from build123d import *

# Parameters (mm, degrees)
BOSS_EXTRUDE2_DEPTH = 6
BOSS_EXTRUDE4_DEPTH = 12
CUT_EXTRUDE4_DEPTH  = 56.306509563
FILLET3_R           = 5
FILLET7_R           = 2
FILLET4_R           = 2
FILLET5_R           = 0.5
FILLET6_R           = 1


with BuildPart() as part:
    # Sketch1 → Boss-Extrude2 (new body)
    with BuildSketch(Plane(origin=(0, 0, 0), x_dir=(1, 0, 0), z_dir=(0, 1, 0))):
        Polygon((13, 5), (-13, 5), (-13, 16), (-25.45, 16), (-25.45, 0), (25.45, 0), (25.45, 16), (13, 16), align=None)
        with BuildLine():
            ThreePointArc((-19.547918472, 10.202081528), (-20.75, 7.3), (-21.952081528, 10.202081528))
            Line((-21.952081528, 10.202081528), (-20.75, 11.404163056))
            Line((-20.75, 11.404163056), (-19.547918472, 10.202081528))
        make_face(mode=Mode.SUBTRACT)
        with BuildLine():
            Line((20.75, 11.404163056), (21.952081528, 10.202081528))
            ThreePointArc((21.952081528, 10.202081528), (20.75, 7.3), (19.547918472, 10.202081528))
            Line((19.547918472, 10.202081528), (20.75, 11.404163056))
        make_face(mode=Mode.SUBTRACT)
    extrude(amount=BOSS_EXTRUDE2_DEPTH)

    # Sketch1<4> → Boss-Extrude4 (add)
    with BuildSketch(Plane(origin=(0, 0, 0), x_dir=(1, 0, 0), z_dir=(0, 1, 0))):
        Polygon((25.45, 0), (-25.45, 0), (-25.45, -18), (-20.45, -18), (-20.45, -3), (9.55, -3), (9.55, -18), (14.55, -18), (14.55, -3), (25.45, -3), align=None)
    extrude(amount=BOSS_EXTRUDE4_DEPTH)

    # Sketch9 → Cut-Extrude4 (cut, through all)
    with BuildSketch(Plane.ZY.offset(25.45)):
        with BuildLine():
            Line((9.378679656, 8.121320344), (11.5, 10.242640687))
            Line((11.5, 10.242640687), (13.621320344, 8.121320344))
            ThreePointArc((13.621320344, 8.121320344), (11.5, 3), (9.378679656, 8.121320344))
        make_face()
    extrude(amount=-CUT_EXTRUDE4_DEPTH, mode=Mode.SUBTRACT)

    # Fillet3
    fillet3_edges = [part.edges().sort_by_distance(p)[0] for p in [
        (-22.95, 12, 18),
        (12.05, 12, 18),
    ]]
    fillet(fillet3_edges, radius=FILLET3_R)

    # Fillet7
    fillet7_edges = [part.edges().sort_by_distance(p)[0] for p in [
        (-5.45, 0, 3),
    ]]
    fillet(fillet7_edges, radius=FILLET7_R)

    # Fillet4
    # the kernel refuses this fillet: 2 mm, written as the material it adds along each edge
    with BuildSketch(Plane(origin=(9.55, 2, 1), x_dir=(0, 0.8017442392976483, -0.5976672776328277), z_dir=(0, 0.5976672776328277, 0.8017442392976483))) as fillet4_piece_1_section:
        with BuildLine():
            CenterArc((2 + FILLET4_R, FILLET4_R), FILLET4_R, 180, 90)
            Line((2, FILLET4_R), (2, 0))
            Line((2, 0), (2 + FILLET4_R, 0))
        make_face()
    fillet4_piece_1 = revolve(axis=Axis((9.55, 2, 1), (-1, 0, 0)), revolution_arc=233.296989237, mode=Mode.PRIVATE)
    fillet4_piece_1 = split(fillet4_piece_1, bisect_by=Plane(origin=(8.926743459, 0, 2.499877942), z_dir=(0, 1, 0)), keep=Keep.TOP, mode=Mode.PRIVATE)
    add(fillet4_piece_1)
    with BuildSketch(Plane(origin=(-20.45, 2, 1), x_dir=(0, 0.8017442392976483, -0.5976672776328277), z_dir=(0, 0.5976672776328277, 0.8017442392976483))) as fillet4_piece_2_section:
        with BuildLine():
            CenterArc((2 + FILLET4_R, -FILLET4_R), FILLET4_R, 90, 90)
            Line((2 + FILLET4_R, 0), (2, 0))
            Line((2, 0), (2, -FILLET4_R))
        make_face()
    fillet4_piece_2 = revolve(axis=Axis((-20.45, 2, 1), (-1, 0, 0)), revolution_arc=233.296989237, mode=Mode.PRIVATE)
    fillet4_piece_2 = split(fillet4_piece_2, bisect_by=Plane(origin=(-19.826743524, 0, 2.499877995), z_dir=(0, 1, 0)), keep=Keep.TOP, mode=Mode.PRIVATE)
    add(fillet4_piece_2)
    with BuildSketch(Plane(origin=(14.55, 0, 3), x_dir=(1, 0, 0), z_dir=(0, 1, 0))) as fillet4_piece_3:
        with BuildLine():
            CenterArc((FILLET4_R, -FILLET4_R), FILLET4_R, 90, 90)
            Line((0, -FILLET4_R), (0, 0))
            Line((0, 0), (FILLET4_R, 0))
        make_face()
    extrude(amount=12)
    with BuildSketch(Plane(origin=(-20.45, 2, 3), x_dir=(1, 0, 0), z_dir=(0, 1, 0))) as fillet4_piece_4:
        with BuildLine():
            CenterArc((FILLET4_R, -FILLET4_R), FILLET4_R, 90, 90)
            Line((0, -FILLET4_R), (0, 0))
            Line((0, 0), (FILLET4_R, 0))
        make_face()
    extrude(amount=10)
    with BuildSketch(Plane(origin=(9.55, 2, 3), x_dir=(-1, 0, 0), z_dir=(0, 1, 0))) as fillet4_piece_5:
        with BuildLine():
            CenterArc((FILLET4_R, FILLET4_R), FILLET4_R, 180, 90)
            Line((0, FILLET4_R), (0, 0))
            Line((0, 0), (FILLET4_R, 0))
        make_face()
    extrude(amount=10)

    # Fillet5
    fillet5_edges = [part.edges().sort_by_distance(p)[0] for p in [
        (0, 6, 0),
    ]]
    fillet(fillet5_edges, radius=FILLET5_R)

    # Fillet6
    fillet6_edges = [part.edges().sort_by_distance(p)[0] for p in [
        (-25.45, 3, -16),
        (-13, 3, -16),
        (13, 3, -16),
        (25.45, 3, -16),
        (25.45, 6, 3),
        (-22.95, 0, 18),
        (12.05, 0, 18),
    ]]
    fillet(fillet6_edges, radius=FILLET6_R)


solid = part.part
Could you check a few things on this model? Use its own coordinates, in mm. A direction names the side the tool comes from. Give positions to 0.01 mm unless a question says otherwise; leave off trailing zeros. Write each loop counter-clockwise with the first axis right and the second up, starting at its lowest first coordinate (ties: lowest second). Pieces come first, ordered by that corner, then holes. Notation, with made-up numbers: (-33, 71.25) -> (21, 71.25) arc R25 ccw to (21, 99.25) -> close; hole circle Ø1 at (23.25, 82.25). An arc over 180 degrees is marked (long way). Answer as CSV lines item,"result". Start each with the question number.
(1) Which directions (+Z, -Z, +X, -X, +Y, -Y) give clear straight access to the entire face, cutting with the end or side of a thin tool? Please do faces 4 (the face through (0, 9, 0)), 5 (the face through (-19.85, 6.93, 3.57)), 6 (the face through (-20.157, 2.958, -10.812)), 7 (the face through (13, 3, -10)), 8 (the face through (-25.45, 5, 1)).
(2) If we mould it in two halves opening along Y, with no side actions, what happens to faces 1 (the face through (0, 6, -3)), 2 (the face through (12, 3, 11.6)), 3 (the face through (20, 6, 3))? For each: +Y half, -Y half, draft (parallel to the pull), parting line (faces both ways), or undercut.
(3) If we section it at C-C, the plane x = -3: Write out the boundary of the cut face in (y, z), and give its area (3 significant figures).
(4) Please list where these lines run through material, in increasing order: line 1 (X direction, y = 4, z = -9); line 2 (X direction, y = 7.75, z = 17.5); line 3 (Z direction, x = -17.5, y = 9).
(5) If we section it at B-B, the plane z = 16: Write out the boundary of the cut face in (x, y).
(6) I'm going to push flat-ended pins straight in: pin 1 Ø8 at (x, z) = (12, -11.5) entering from +Y; pin 2 Ø5 at (x, y) = (-0.5, 6.5) entering from +Z; pin 3 Ø1.6 at (x, y) = (3.5, 10) entering from -Z. Where does each tip first touch, or does it pass through?
(7) If we section it at D-D, the plane y = 8.75: Write out the boundary of the cut face in (x, z).
(8) If we section it at A-A, the plane z = -9: Write out the boundary of the cut face in (x, y), and give its area (3 significant figures).
Answer list:
1,face 4,"-Z, +X, -X, +Y"
1,face 5,"+Z, +Y, -Y"
1,face 6,"+Y, -Y"
1,face 7,"-Z, +Y, -Y"
1,face 8,"+Z, -Z, -X, +Y, -Y"
2,face 1,"+Y half"
2,face 2,"undercut"
2,face 3,"draft"
3,outline,"(0, -5) -> (6, -5) -> (6, -0.5) arc R0.5 cw to (6.5, 0) -> (12, 0) -> (12, 3) -> (2, 3) arc R2 ccw to (0, 1) -> close"
3,area,"65.2 mm^2"
4,line 1,"-25.45 to -22.45, -19.05 to -13, 13 to 19.05, 22.45 to 25.45"
4,line 2,"-25.45 to -20.45, 9.55 to 14.55"
4,line 3,"0 to 3"
5,outline,"(-25.45, 0) -> (-20.45, 0) -> (-20.45, 11) -> (-25.45, 11) -> close; (9.55, 0) -> (14.55, 0) -> (14.55, 11) -> (9.55, 11) -> close"
6,pin 1,"y = 6"
6,pin 2,"z = 3"
6,pin 3,"z = 0"
7,outline,"(-25.45, 0) -> (25.45, 0) -> (25.45, 2) arc R1 ccw to (24.45, 3) -> (16.55, 3) arc R2 cw to (14.55, 5) -> (14.55, 10.01) -> (9.55, 10.01) -> (9.55, 5) arc R2 cw to (7.55, 3) -> (-18.45, 3) arc R2 cw to (-20.45, 5) -> (-20.45, 10.01) -> (-25.45, 10.01) -> close; (-25.45, 12.99) -> (-20.45, 12.99) -> (-20.45, 17.68) -> (-25.45, 17.68) -> close; (9.55, 12.99) -> (14.55, 12.99) -> (14.55, 17.68) -> (9.55, 17.68) -> close"
8,outline,"(-25.45, 0) -> (-22.45, 0) -> (-22.45, 6) -> (-25.45, 6) -> close; (-19.05, 0) -> (-13, 0) -> (-13, 6) -> (-19.05, 6) -> close; (13, 0) -> (19.05, 0) -> (19.05, 6) -> (13, 6) -> close; (22.45, 0) -> (25.45, 0) -> (25.45, 6) -> (22.45, 6) -> close"
8,area,"109 mm^2"
